Geometry: final body of the model. Coordinates: model frame, mm. Face numbers are marked on the shaded views. A direction names the side the tool comes from. Give positions to 0.01 mm unless a question says otherwise; leave off trailing zeros. Order: outer loops, then holes, each group sorted by start corner. A loop starts at its lowest first (then second) coordinate and runs counter-clockwise, first axis right, second up. Notation, with made-up numbers: (27, -22) - (81, -22) arc R16 cw to (81, -9) - close; hole circle Ø6 at (18.5, 58.5). An arc over 180 degrees is marked (long way). One line per question, with ' | ' between items. Start each with the question number.
from build123d import *

# Parameters (mm, degrees)
SKETCH1_W            = 100
SKETCH1_H            = 200
BOSS_EXTRUDE1_DEPTH  = 25
BOSS_EXTRUDE3_REACH  = 224.221
SKETCH4_R            = 12.5
BOSS_EXTRUDE4_DEPTH  = 15
SKETCH5_R            = 6
CUT_EXTRUDE1_DEPTH   = 225.303099777
SKETCH6_W            = 100
SKETCH6_H            = 37.5
BOSS_EXTRUDE5_DEPTH  = 10
SKETCH7_W            = 100
SKETCH7_H            = 37.5
BOSS_EXTRUDE6_DEPTH  = 10
SKETCH8_W            = 100
SKETCH8_H            = 60
BOSS_EXTRUDE7_DEPTH  = 15
BOSS_EXTRUDE9_DEPTH  = 37
SKETCH12_R           = 7.5
CUT_EXTRUDE7_DEPTH   = 5
CUT_EXTRUDE8_DEPTH   = 5
CUT_EXTRUDE9_DEPTH   = 5
BOSS_EXTRUDE10_DEPTH = 30
CUT_EXTRUDE10_DEPTH  = 30
SKETCH18_R           = 5
CUT_EXTRUDE11_DEPTH  = 206.831491767


with BuildPart() as part:
    # Sketch1 → Boss-Extrude1 (new body)
    with BuildSketch(Plane(origin=(0, 0, 0), x_dir=(1, 0, 0), z_dir=(0, 1, 0))):
        with Locations((50, -100)):
            Rectangle(SKETCH1_W, SKETCH1_H)
    extrude(amount=BOSS_EXTRUDE1_DEPTH)

    # Boss-Extrude3: up to this face of the body (flat: up to its plane)
    boss_extrude3_end = Plane(part.part.faces().sort_by_distance((50, 0, 100))[0])
    # Sketch3 → Boss-Extrude3 (add, up to the picked face)
    with BuildSketch(Plane(origin=(19.732622965, 54.214936023, 0), x_dir=(0, 0, -1), z_dir=(0.34202014332566943, 0.9396926207859081, 0)), mode=Mode.PRIVATE) as boss_extrude3_sk1:
        with BuildLine():
            Line((-185, -85.418758495), (-135, -85.418758495))
            Line((-135, -85.418758495), (-135, -45.418758495))
            ThreePointArc((-135, -45.418758495), (-160, -20.418758495), (-185, -45.418758495))
            Line((-185, -45.418758495), (-185, -85.418758495))
        make_face()
    boss_extrude3_tool1 = split(extrude(boss_extrude3_sk1.sketch, amount=-BOSS_EXTRUDE3_REACH, mode=Mode.PRIVATE), bisect_by=boss_extrude3_end, keep=Keep.BOTH, mode=Mode.PRIVATE)
    add(boss_extrude3_tool1.solids().sort_by(Axis((71.735431, 35.287462, 160), (-0.34202014332566943, -0.9396926207859081, 0)))[0])

    # Sketch4 → Boss-Extrude4 (add)
    with BuildSketch(Plane(origin=(19.732622965, 54.214936023, 0), x_dir=(0.9396926207859082, -0.34202014332566943, 0), z_dir=(0.34202014332566943, 0.9396926207859082, 0))):
        with Locations(Location((45.418758495, -160, 0), (0, 0, 180))):
            Circle(SKETCH4_R)
    extrude(amount=BOSS_EXTRUDE4_DEPTH)

    # Sketch5 → Cut-Extrude1 (cut, through all)
    with BuildSketch(Plane(origin=(24.862925115, 68.310325335, 0), x_dir=(0.9396926207859082, -0.34202014332566943, 0), z_dir=(0.34202014332566943, 0.9396926207859082, 0))):
        with Locations(Location((45.418758495, -160, 0), (0, 0, 180))):
            Circle(SKETCH5_R)
    extrude(amount=-CUT_EXTRUDE1_DEPTH, mode=Mode.SUBTRACT)

    # Sketch6 → Boss-Extrude5 (add)
    with BuildSketch(Plane.XZ):
        with Locations((50, 131.25)):
            Rectangle(SKETCH6_W, SKETCH6_H)
    extrude(amount=BOSS_EXTRUDE5_DEPTH)

    # Sketch7 → Boss-Extrude6 (add)
    with BuildSketch(Plane.XZ):
        with Locations((50, 68.75)):
            Rectangle(SKETCH7_W, SKETCH7_H)
    extrude(amount=BOSS_EXTRUDE6_DEPTH)

    # Sketch8 → Boss-Extrude7 (add)
    with BuildSketch(Plane(origin=(0, 25, 0), x_dir=(1, 0, 0), z_dir=(0, 1, 0))):
        with Locations((50, -30)):
            Rectangle(SKETCH8_W, SKETCH8_H)
    extrude(amount=BOSS_EXTRUDE7_DEPTH)

    # Sketch10 → Boss-Extrude9 (add)
    with BuildSketch(Plane(origin=(0, 62.051270189, 35.825317547), x_dir=(1, 0, 0), z_dir=(0, 0.866025403784438, 0.500000000000001))):
        with BuildLine():
            Line((0, -74.102540378), (70, -74.102540378))
            Line((70, -74.102540378), (70, -24.102540378))
            ThreePointArc((70, -24.102540378), (35, 10.897459622), (0, -24.102540378))
            Line((0, -24.102540378), (0, -74.102540378))
        make_face()
    extrude(amount=-BOSS_EXTRUDE9_DEPTH)

    # Sketch12 → Cut-Extrude7 (cut)
    with BuildSketch(Plane(origin=(0, 62.051270189, 35.825317547), x_dir=(1, 0, 0), z_dir=(0, 0.8660254037844382, 0.500000000000001))):
        with Locations(Location((35, -24.102540378, 0), (0, 0, 270))):
            Circle(SKETCH12_R)
    extrude(amount=-CUT_EXTRUDE7_DEPTH, mode=Mode.SUBTRACT)

    # Sketch13 → Cut-Extrude8 (cut)
    with BuildSketch(Plane(origin=(0, 62.051270189, 35.825317547), x_dir=(1, 0, 0), z_dir=(0, 0.8660254037844382, 0.500000000000001))):
        with BuildLine():
            Line((35, -74.102540378), (40, -74.102540378))
            Line((40, -74.102540378), (40, -29.507888224))
            ThreePointArc((40, -29.507888224), (35, -31.465813111), (30, -29.507888224))
            Line((30, -29.507888224), (30, -74.102540378))
            Line((30, -74.102540378), (35, -74.102540378))
        make_face()
        with BuildLine():
            Line((40, -18.697192533), (40, 10.538475773))
            ThreePointArc((40, 10.538475773), (35, 10.897459622), (30, 10.538475773))
            Line((30, 10.538475773), (30, -18.697192533))
            ThreePointArc((30, -18.697192533), (35, -16.739267646), (40, -18.697192533))
        make_face()
    extrude(amount=-CUT_EXTRUDE8_DEPTH, mode=Mode.SUBTRACT)

    # Sketch14 → Cut-Extrude9 (cut)
    with BuildSketch(Plane(origin=(0, 62.051270189, 35.825317547), x_dir=(1, 0, 0), z_dir=(0, 0.8660254037844382, 0.500000000000001))):
        with BuildLine():
            Line((29.409830056, -19.102540378), (0.181014248, -19.102540378))
            ThreePointArc((0.181014248, -19.102540378), (-0.176153411, -24.102540378), (0.181014248, -29.102540378))
            Line((0.181014248, -29.102540378), (29.409830056, -29.102540378))
            ThreePointArc((29.409830056, -29.102540378), (27.5, -24.102540378), (29.409830056, -19.102540378))
        make_face()
        with BuildLine():
            Line((40.590169944, -19.102540378), (69.818985752, -19.102540378))
            ThreePointArc((69.818985752, -19.102540378), (70.176153411, -24.102540378), (69.818985752, -29.102540378))
            Line((69.818985752, -29.102540378), (40.590169944, -29.102540378))
            ThreePointArc((40.590169944, -29.102540378), (42.5, -24.102540378), (40.590169944, -19.102540378))
        make_face()
    extrude(amount=-CUT_EXTRUDE9_DEPTH, mode=Mode.SUBTRACT)

    # Sketch16 → Boss-Extrude10 (add)
    with BuildSketch(Plane(origin=(100, 0, 0), x_dir=(0, 0, -1), z_dir=(1, 0, 0))):
        with BuildLine():
            Line((-121.794494718, 25), (-200, 25))
            Line((-200, 25), (-200, 0))
            Line((-200, 0), (-150, 0))
            Line((-150, 0), (-150, -10))
            Line((-150, -10), (-112.5, -10))
            Line((-112.5, -10), (-112.5, 0))
            Line((-112.5, 0), (-87.5, 0))
            Line((-87.5, 0), (-87.5, -10))
            Line((-87.5, -10), (-50, -10))
            Line((-50, -10), (-50, 0))
            Line((-50, 0), (0, 0))
            Line((0, 0), (0, 40))
            Line((0, 40), (-60, 40))
            ThreePointArc((-60, 40), (-88.205505282, 21.411010565), (-121.794494718, 25))
        make_face()
    extrude(amount=-BOSS_EXTRUDE10_DEPTH)

    # Sketch17 → Cut-Extrude10 (cut)
    with BuildSketch(Plane(origin=(100, 0, 0), x_dir=(0, 0, -1), z_dir=(1, 0, 0))):
        with BuildLine():
            Line((-121.794494718, 25), (-78.205505282, 25))
            ThreePointArc((-78.205505282, 25), (-100, 20), (-121.794494718, 25))
        make_face()
    extrude(amount=-CUT_EXTRUDE10_DEPTH, mode=Mode.SUBTRACT)

    # Sketch18 → Cut-Extrude11 (cut, through all)
    with BuildSketch(Plane(origin=(0, 57.72114317, 33.325317547), x_dir=(1, 0, 0), z_dir=(0, 0.8660254037844382, 0.5000000000000011))):
        with Locations(Location((35, -24.102540378, 0), (0, 0, 270))):
            Circle(SKETCH18_R)
    extrude(amount=-CUT_EXTRUDE11_DEPTH, mode=Mode.SUBTRACT)


solid = part.part
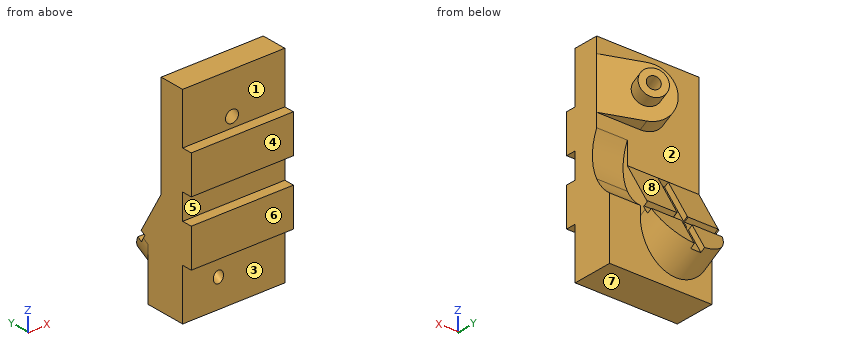
(1) Cut plane B-B, the plane x = 10. Return the cut outline in (y, z).
(2) Cut plane C-C, the plane z = 131. Return the cut outline in (x, y), plus the area to 3 significant figures.
(3) Cut plane A-A, the plane y = 32.5. Give the number of separate pieces and of enclosed holes in the cut face, plus the area to 3 significant figures.
(4) Material intervals for line 1 along Z through (x, y) = (65.5, 49); line 2 along Y through (x, z) = (51, 142.5); line 3 along Z through (x, y) = (75.5, -5), sorted ascending. Write a range as from..to.
(5) Access query for the marked faces 1, 2, 3, 4 and 5. Directions: +Z, -Z, +X, -X, +Y, -Y. A direction counts if a zero-diameter tool reaches every point of the face in a straight line with its end or side. Return the directions, or none.
(6) Contact query for flat-ended pins moving along their axis: P1, Ø4, axis at x = 82, z = 100.5, coming from the +Y side; P2, Ø1.5, axis at x = 58.5, y = 43, coming from the -Z side; P3, Ø4, axis at y = 28.5, z = 152.5, coming from the -X side; P4, Ø8, axis at x = 36, y = -3.5, coming from the -Z side. Output: stop coordinate, or through.
(7) Pull-direction query (Z, two-part tool) for the marked faces 6, 7 and 8; classes: +Z half, -Z half, draft (parallel to the pull), parting line (faces both ways), or undercut.
(8) Cut plane D-D, the plane x = 84.5. Return the cut outline in (y, z), plus the area to 3 significant figures.
Results are:
1) outline: (-10, 50) - (0, 50) - (0, 0) - (40, 0) - (40, 22.64) - (62.25, 35.49) - (52.5, 52.37) - (48.17, 49.87) - (43.17, 58.53) - (47.5, 61.03) - (25, 100) - (25, 200) - (0, 200) - (0, 150) - (-10, 150) - (-10, 112.5) - (0, 112.5) - (0, 87.5) - (-10, 87.5) - close
2) outline: (0, -10) - (100, -10) - (100, 25) - (0, 25) - close | area: 3,500 mm2
3) separate pieces: 2 | enclosed holes: 2 | area: 9,790 mm2
4) line 1: 36.3..50.35, 147.52..154.03, 165.97..172.48 | line 2: -10..42.83 | line 3: 50..87.5, 112.5..150
5) face 1: +Z, +X, -X, -Y | face 2: -X, +Y | face 3: -Z, +X, -X, -Y | face 4: +Z, -Z, +X, -X, -Y | face 5: +X, -X, -Y
6) P1: y = 20.06 | P2: z = 21.83 | P3: x = 32.38 | P4: z = 0
7) face 6: draft | face 7: -Z half | face 8: undercut
8) outline: (-10, 50) - (0, 50) - (0, 0) - (40, 0) - (40, 60) arc R50 cw to (25, 121.79) - (25, 135) - (30.64, 135) - (30.64, 185) - (25, 185) - (25, 200) - (0, 200) - (0, 150) - (-10, 150) - (-10, 112.5) - (0, 112.5) - (0, 87.5) - (-10, 87.5) - close | area: 6,900 mm2
